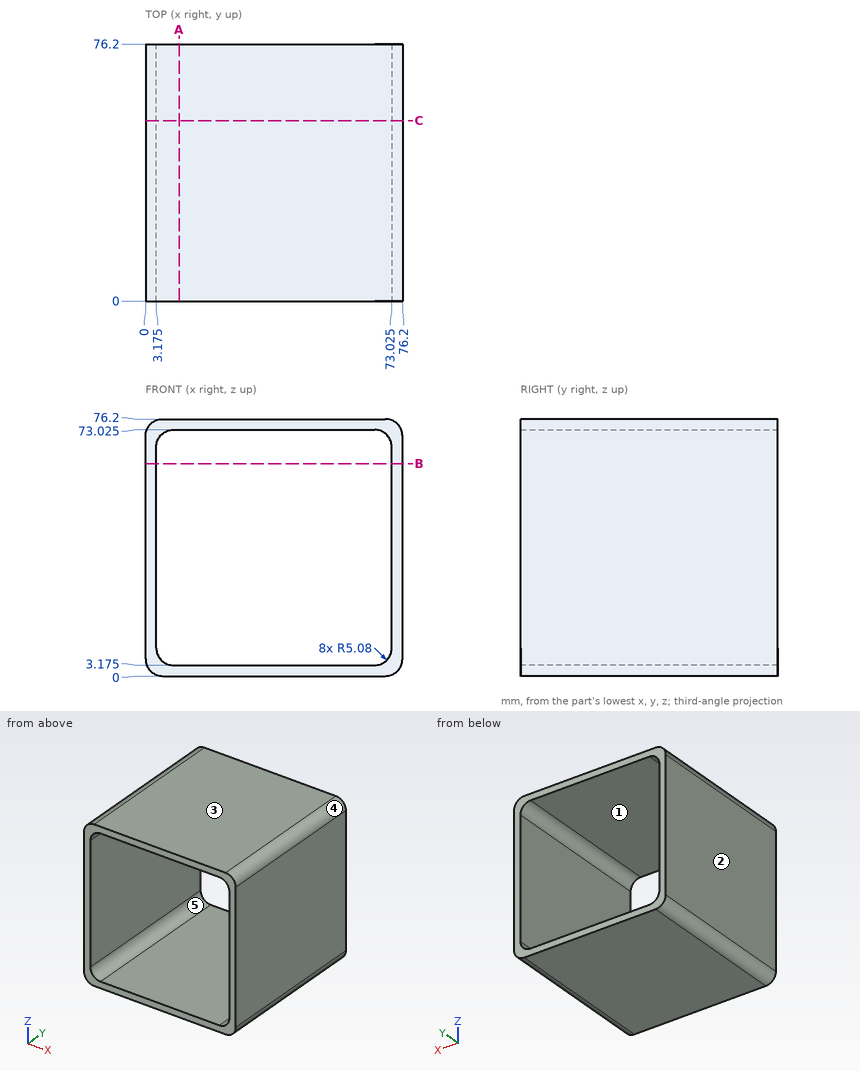
Check sheet for the drawn part. Datum: minimum x, y, z corner. Units: mm. A direction names the side the tool comes from. Give positions to 0.01 mm unless a question says otherwise; leave off trailing zeros. Write each loop counter-clockwise with the first axis right and the second up, starting at its lowest first coordinate (ties: lowest second). Pieces come first, ordered by that corner, then holes.
(1) Access from +Z, -Z, +X, -X, +Y, -Y to the whole of each face (thin tool, end or side, straight path). Record for the marked faces 4 and 5.
(2) Gauge pin test, flat end, axial feed: pin 1 (12 mm diameter, centred on x = 45.5, z = 8.5, fed in from -Y). Record the tip position at first contact, or that the pin passes through.
(3) Cross-section at A-A (x = 10). Enter the section's corners in (y, z) (3 decimals).
(4) Cross-section at B-B (z = 63). Enter the section's corners in (x, y) (3 decimals), plus the area to 3 significant figures.
(5) Mould release check, pull along X, two halves, no side actions. Record for the marked faces 1, 2 and 3: +X half, -X half, draft (parallel to the pull), parting line (faces both ways), or undercut.
(6) Cross-section at C-C (y = 53.5). Enter the section's corners in (x, z) (3 decimals).
(7) Material ranges on line 1 (X direction, y = 16.5, z = 40) (3 decimals); line 2 (X direction, y = 8, z = 71), recorded low to high.
Worked out:
1. face 4: +Z, +X, +Y, -Y
1. face 5: +Y, -Y
2. pin 1: stops at y = 0
3. outline: (0, 0) - (76.2, 0) - (76.2, 3.175) - (0, 3.175) - close; (0, 73.025) - (76.2, 73.025) - (76.2, 76.2) - (0, 76.2) - close
4. outline: (0, 0) - (3.175, 0) - (3.175, 76.2) - (0, 76.2) - close; (73.025, 0) - (76.2, 0) - (76.2, 76.2) - (73.025, 76.2) - close
4. area: 484 mm2
5. face 1: undercut
5. face 2: -X half
5. face 3: draft
6. outline: (0, 5.08) arc R5.08 ccw to (5.08, 0) - (71.12, 0) arc R5.08 ccw to (76.2, 5.08) - (76.2, 71.12) arc R5.08 ccw to (71.12, 76.2) - (5.08, 76.2) arc R5.08 ccw to (0, 71.12) - close; hole (3.175, 8.255) arc R5.08 ccw to (8.255, 3.175) - (67.945, 3.175) arc R5.08 ccw to (73.025, 8.255) - (73.025, 67.945) arc R5.08 ccw to (67.945, 73.025) - (8.255, 73.025) arc R5.08 ccw to (3.175, 67.945) - close
7. line 1: x = 0 to 3.175, 73.025 to 76.2
7. line 2: x = 0 to 4.2, 72 to 76.2
